Could you check a few things on this model? Use its own coordinates, in mm. Face numbers are marked on the shaded views. A direction names the side the tool comes from. Give positions to 0.01 mm unless a question says otherwise; leave off trailing zeros. Order: outer loops, then holes, each group sorted by start corner. A loop starts at its lowest first (then second) coordinate and runs counter-clockwise, first axis right, second up. Notation, with made-up numbers: M 4,64 L 39,64 A28 cw 39,93 Z; hole C -19.75,24.25 d9. An arc over 180 degrees is marked long. Use a Markdown table: item, result. Add a question column.
Item 1: If we mould it in two halves opening along Y, with no side actions, what happens to the marked faces 1, 2, 3 and 4? For each: released by +Y, released by -Y, zero draft, split by the parting line, or undercut.
Item 2: Suppose I cut it at C-C on z = -2.5. Write out the boundary of the cut face in (x, y), plus the area to 3 significant figures.
Item 3: I'm going to push flat-ended pins straight in: pin 1 Ø2.5 at (y, z) = (8, -7.5) entering from -X; pin 2 Ø3 at (y, z) = (-9.5, -1) entering from -X; pin 3 Ø6.5 at (y, z) = (-8, -7.5) entering from -X; pin 4 Ø13 at (x, y) = (0, 0) entering from +Z. Where does each tip first touch, or does it pass through?
Item 4: Suppose I cut it at D-D on y = 4. Write out the boundary of the cut face in (x, z).
Item 5: For the marked faces 5, 6 and 7, which set-ups out of +Z, -Z, +X, -X, +Y, -Y let a thin tool reach every point of the face, with its end or its side?
Item 6: Suppose I cut it at A-A on y = 0. Write out the boundary of the cut face in (x, z), plus the area to 3 significant figures.
Item 7: If I drill on L1, parallel to X at y = 0, z = 3.75; L2, parallel to X at y = 11, z = -13; L3, parallel to Z at x = -11, y = 9, over which ranges is the centre line in solid material (lowest first)? Write a range as from..to.
Item 8: Suppose I cut it at B-B on x = 1.5. Write out the boundary of the cut face in (y, z).
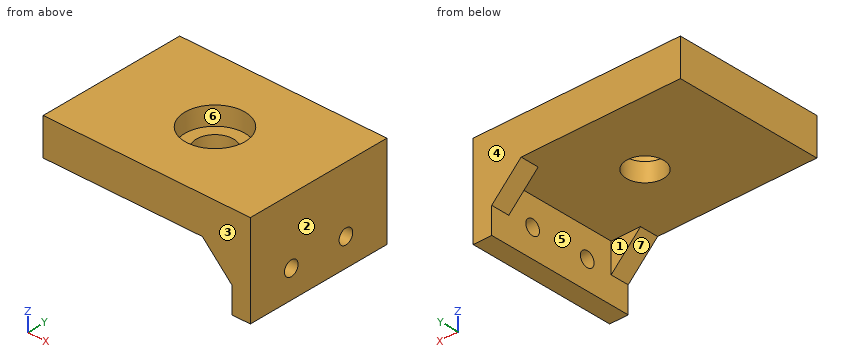
from build123d import *

# Parameters (mm, degrees)
SKETCH1_W           = 55.88
SKETCH1_H           = 40
SKETCH1_R           = 5
BOSS_EXTRUDE1_DEPTH = 10
SKETCH2_R           = 8.1
CUT_EXTRUDE1_DEPTH  = 5
SKETCH3_W           = 5
SKETCH3_H           = 40
BOSS_EXTRUDE3_DEPTH = 15
RIB1_REACH          = 53.046
SKETCH4_WALL_W      = 115.312280144
SKETCH4_WALL_H      = 5
SKETCH5_R           = 2
CUT_EXTRUDE2_DEPTH  = 15


with BuildPart() as part:
    # Sketch1 → Boss-Extrude1 (new body)
    with BuildSketch(Plane.XY):
        Rectangle(SKETCH1_W, SKETCH1_H)
        Circle(SKETCH1_R, mode=Mode.SUBTRACT)
    extrude(amount=BOSS_EXTRUDE1_DEPTH)

    # Sketch2 → Cut-Extrude1 (cut)
    with BuildSketch(Plane.XY.offset(10)):
        Circle(SKETCH2_R)
    extrude(amount=-CUT_EXTRUDE1_DEPTH, mode=Mode.SUBTRACT)

    # Sketch3 → Boss-Extrude3 (add)
    with BuildSketch(Plane(origin=(0, 0, 0), x_dir=(-1, 0, 0), z_dir=(0, 0, -1))):
        with Locations((-25.44, 0)):
            Rectangle(SKETCH3_W, SKETCH3_H)
    extrude(amount=BOSS_EXTRUDE3_DEPTH)

    # Sketch4 wall → Rib1 (add, up to next)
    with BuildSketch(Plane(origin=(18.972682027, 20, -3.967317973), x_dir=(0.707106781187, 0, -0.707106781187), z_dir=(-0.707106781187, 0, -0.707106781187)), mode=Mode.PRIVATE) as rib1_sk1:
        with Locations((0, 2.5)):
            Rectangle(SKETCH4_WALL_W, SKETCH4_WALL_H)
    rib1_tool1 = extrude(rib1_sk1.sketch, amount=-RIB1_REACH, mode=Mode.PRIVATE) - part.part
    rib1 = rib1_tool1.solids().sort_by_distance((18.972682027, 20, -3.967317973))[0]
    add(rib1)

    # Mirror1: Rib1 across plane
    add(rib1.mirror(Plane.ZX))

    # Sketch5 → Cut-Extrude2 (cut)
    with BuildSketch(Plane.ZY.offset(-22.94)):
        with Locations(Location((-7.5, 8, 0), (0, 0, 270))):
            Circle(SKETCH5_R)
        with Locations((-7.5, -8)):
            Circle(SKETCH5_R)
    extrude(amount=-CUT_EXTRUDE2_DEPTH, mode=Mode.SUBTRACT)


solid = part.part
Findings below:
| question | item | result |
|---|---|---|
| 1 | face 1 | undercut |
| 1 | face 2 | zero draft |
| 1 | face 3 | released by -Y |
| 1 | face 4 | released by +Y |
| 2 | outline | M 17.51,-20 L 27.94,-20 L 27.94,20 L 17.51,20 L 17.51,15 L 22.94,15 L 22.94,-15 L 17.51,-15 Z |
| 2 | area | 254 mm^2 |
| 3 | pin 1 | passes through |
| 3 | pin 2 | stops at x = -27.94 |
| 3 | pin 3 | stops at x = 22.94 |
| 3 | pin 4 | stops at z = 5 |
| 4 | outline | M -27.94,0 L -3,0 L -3,5 L -7.04,5 L -7.04,10 L -27.94,10 Z; M 3,0 L 22.94,0 L 22.94,-15 L 27.94,-15 L 27.94,10 L 7.04,10 L 7.04,5 L 3,5 Z |
| 5 | face 5 | -Z, -X |
| 5 | face 6 | +Z |
| 5 | face 7 | -Z, -X, +Y, -Y |
| 6 | outline | M -27.94,0 L -5,0 L -5,5 L -8.1,5 L -8.1,10 L -27.94,10 Z; M 5,0 L 22.94,0 L 22.94,-15 L 27.94,-15 L 27.94,10 L 8.1,10 L 8.1,5 L 5,5 Z |
| 6 | area | 503 mm^2 |
| 7 | L1 | x = -27.94..-5, 5..27.94 |
| 7 | L2 | x = 22.94..27.94 |
| 7 | L3 | z = 0..10 |
| 8 | outline | M -20,0 L -4.77,0 L -4.77,5 L -7.96,5 L -7.96,10 L -20,10 Z; M 4.77,0 L 20,0 L 20,10 L 7.96,10 L 7.96,5 L 4.77,5 Z |
